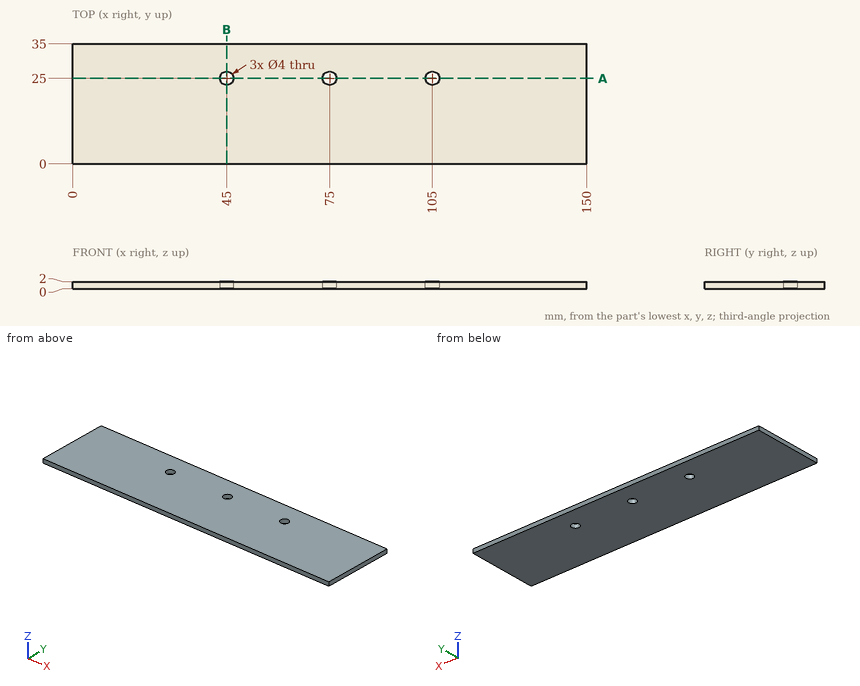
Answer from the drawing. Dimensions are ordinates in mm from the lowest x, y and z of the part. Coordinates: 2 decimals unless noted, no trailing zeros. Write each loop counter-clockwise with the first axis right and the second up, starting at its lowest first coordinate (ties: lowest second). Pieces come first, ordered by that corner, then holes. Notation, with made-up numbers: M -13.5,35.5 L -2.5,35.5 A24 ccw -2.5,52.5 Z; hole C -33.5,-29.5 d5. An arc over 180 degrees is marked long. Put each result on its own line as item: value. Start each with the question number.
1. A cutting plane is placed at B-B on x = 45. Write down the section's boundary in (y, z).
2. A flat-ended cylindrical pin translates along its axis: P1, Ø3.5, axis at x = 45, y = 25, coming from the -Z side. Find the tip coordinate at first contact, or state that the pin passes through.
3. A cutting plane is placed at A-A on y = 25. Write down the section's boundary in (x, z).
4. Consider line 1 (Y direction, x = 105, z = 1.3); line 2 (X direction, y = 26.5, z = 0.95); line 3 (Y direction, x = 43.5, z = 0.1). Determine where each line is inside the solid, lowest interval first. Write a range as from..to.
Resolved:
1. outline: M 0,0 L 23,0 L 23,2 L 0,2 Z; M 27,0 L 35,0 L 35,2 L 27,2 Z
2. P1: passes through
3. outline: M 0,0 L 43,0 L 43,2 L 0,2 Z; M 47,0 L 73,0 L 73,2 L 47,2 Z; M 77,0 L 103,0 L 103,2 L 77,2 Z; M 107,0 L 150,0 L 150,2 L 107,2 Z
4. line 1: y = 0..23, 27..35
4. line 2: x = 0..43.68, 46.32..73.68, 76.32..103.68, 106.32..150
4. line 3: y = 0..23.68, 26.32..35
